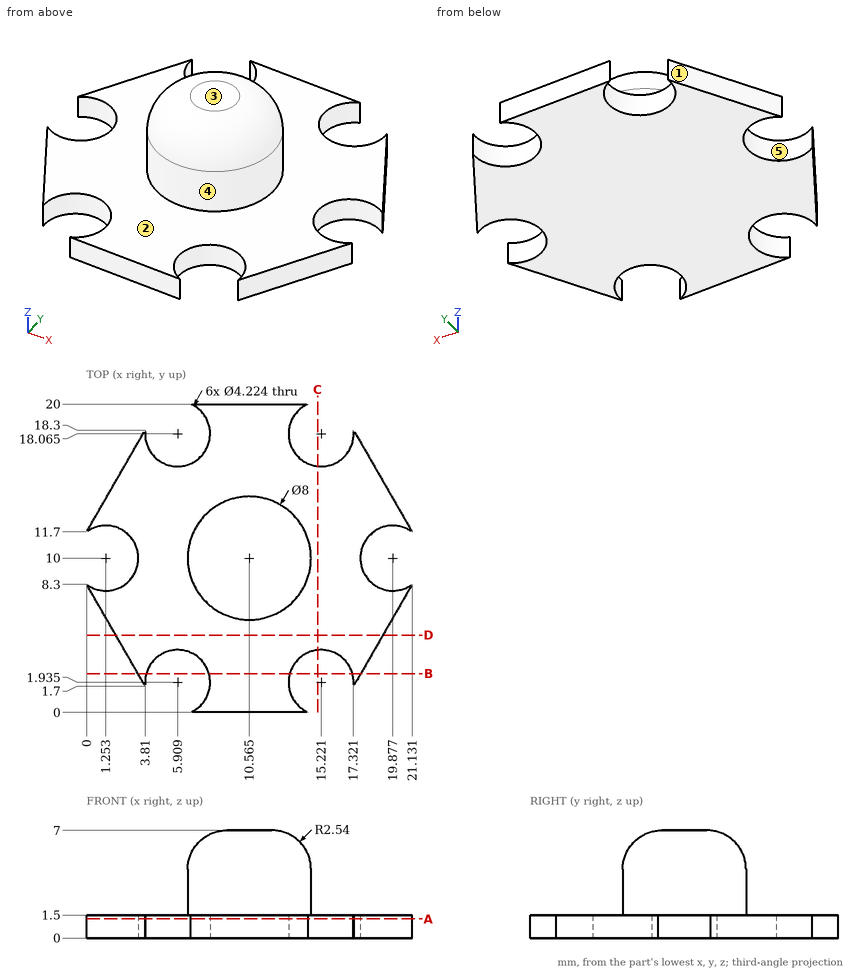
Can you work these out from the drawing? Everything is in mm from the part's minimum corner. A direction names the side the tool comes from. Coordinates: 2 decimals unless noted, no trailing zeros. Loops run counter-clockwise (first coordinate to the right, second up) from the corner with the lowest first, then second, coordinate; pieces in that order, holes last. Notation, with made-up numbers: (69.5, -23.5) -> (111.5, -23.5) arc R17 ccw to (111.5, -10.5) -> close; hole circle Ø11 at (18.5, 27.5). An arc over 180 degrees is marked (long way). Return JSON: item names as keys, results as strings.
1) If we section it at D-D, the plane y = 5: Write out the boundary of the cut face in (x, z) (1 decimal).
Results below:
{"outline": "(1.9, 0) -> (19.2, 0) -> (19.2, 1.5) -> (1.9, 1.5) -> close"}
2) If we section it at C-C, the plane x = 15: Write out the boundary of the cut face in (y, z) (1 decimal).
Results below:
{"outline": "(4, 0) -> (16, 0) -> (16, 1.5) -> (4, 1.5) -> close"}
3) I need wall thicknesses on line 1 (Z direction, x = 5.5, y = 15.5); line 2 (Y direction, x = 19, z = 0.5) (1 decimal); line 3 (Y direction, x = 10.25, z = 3). Which ranges of each line are inside material? Lowest first, please. Write a range as from..to.
Results below:
{"line 1": "0..1.5", "line 2": "4.6..8.1, 11.9..15.4", "line 3": "6.01..13.99"}
4) If we section it at A-A, the plane z = 1.25: Write out the boundary of the cut face in (x, y) (1 decimal).
Results below:
{"outline": "(0, 8.3) -> (3.8, 1.7) arc R2.1 cw (long way) to (6.8, 0) -> (14.4, 0) arc R2.1 cw (long way) to (17.3, 1.7) -> (21.1, 8.3) arc R2.1 cw (long way) to (21.1, 11.7) -> (17.3, 18.3) arc R2.1 cw (long way) to (14.4, 20) -> (6.8, 20) arc R2.1 cw (long way) to (3.8, 18.3) -> (0, 11.7) arc R2.1 cw (long way) to start"}
5) Will these pins go through, and if not, where does the flat tip stop? pin 1 (5 mm diameter, centred on x = 5.91, y = 1.94, fed in from -Z); pin 2 (3.5 mm diameter, centred on x = 15.22, y = 18.06, fed in from +Z); pin 3 (7 mm diameter, centred on x = 19.88, y = 10, fed in from +Z); pin 4 (6 mm diameter, centred on x = 15.5, y = 14.5, fed in from +Z) (1 decimal).
Results below:
{"pin 1": "z = 0", "pin 2": "through", "pin 3": "z = 1.5", "pin 4": "z = 5.7"}
6) Thinking about a two-plate mould opening in X: for the marked faces 3, 4 and 5, which applies, +X half, -X half, draft (parallel to the pull), parting line (faces both ways), or undercut?
Results below:
{"face 3": "draft", "face 4": "parting line", "face 5": "undercut"}
7) For the marked faces 1 and 2, which set-ups out of +Z, -Z, +X, -X, +Y, -Y let a thin tool reach every point of the face, with its end or its side?
Results below:
{"face 1": "+Z, -Z, -X, +Y", "face 2": "+Z"}
8) If we section it at B-B, the plane y = 2.5: Write out the boundary of the cut face in (x, z) (1 decimal).
Results below:
{"outline": "(3.3, 0) -> (3.9, 0) -> (3.9, 1.5) -> (3.3, 1.5) -> close; (7.9, 0) -> (13.2, 0) -> (13.2, 1.5) -> (7.9, 1.5) -> close; (17.3, 0) -> (17.8, 0) -> (17.8, 1.5) -> (17.3, 1.5) -> close"}
